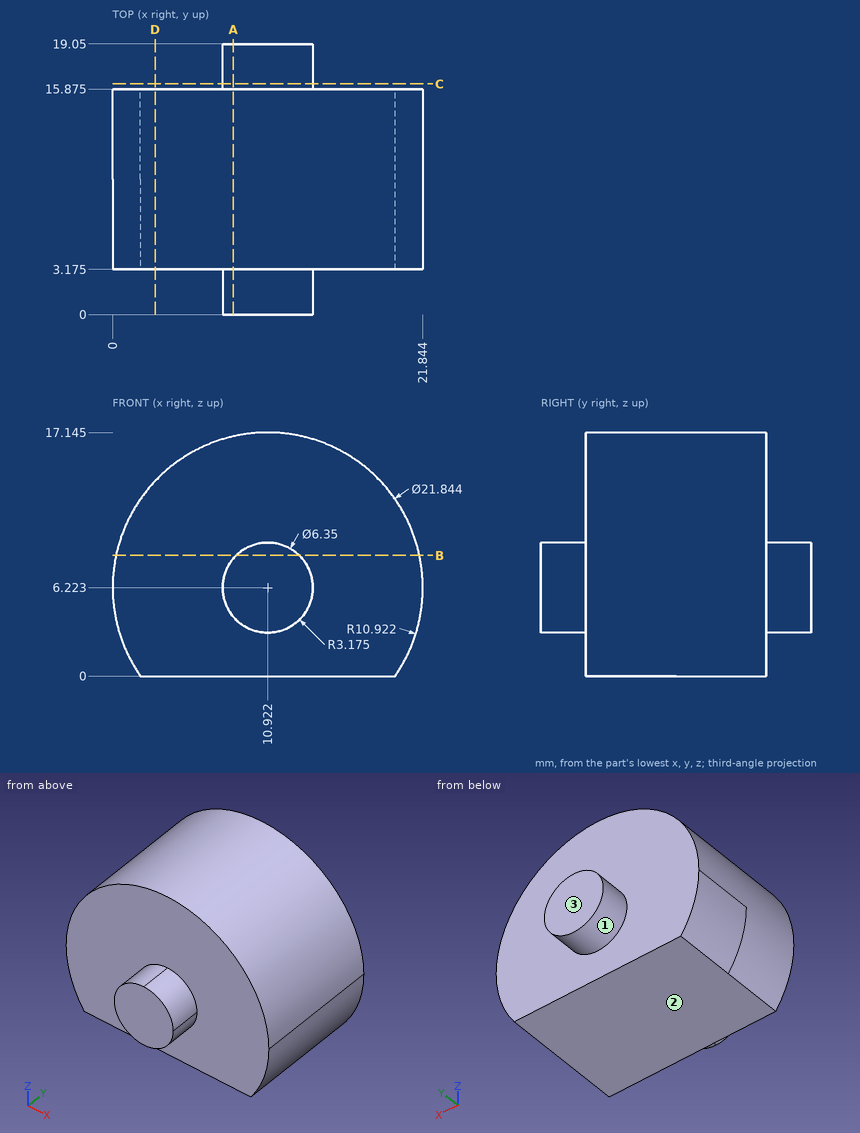
Print and shaded views of the part. All mm, measured from the part's lowest x, y and z. Give positions to 0.01 mm unless a question says otherwise; leave off trailing zeros. Write each loop counter-clockwise with the first axis right and the second up, starting at its lowest first coordinate (ties: lowest second). Pieces come first, ordered by that corner, then holes. Notation, with made-up numbers: (81, 86.5) - (122, 86.5) arc R19 cw to (122, 103.5) - close; hole circle Ø11 at (-33.5, 9.25). An arc over 180 degrees is marked (long way). One line per question, with ' | ' between items. Start each with the question number.
(1) Slice it at B-B on z = 8.5. Write the cut outline in (x, y) (3 decimals), plus the area to 3 significant figures.
(2) Slice it at D-D on x = 3. Write the cut outline in (y, z) (3 decimals), plus the area to 3 significant figures.
(3) Two-plate mould, pull along Z, no slides. Class the marked faces 1, 2 and 3: +Z half, -Z half, draft (parallel to the pull), parting line (faces both ways), or undercut.
(4) Slice it at C-C on y = 16.25. Write the cut outline in (x, z) (3 decimals), plus the area to 3 significant figures.
(5) Wall check: line 1 along Y through (x, z) = (1, 8.75) (3 decimals); line 2 along X through (y, z) = (6.75, 8.5); line 3 along Z through (x, y) = (2.5, 14.25). Give the ranges that are in metal, low to high. Write a range as from..to.
(6) Pin check, flat tips, straight feed: P1, Ø1.5, axis at x = 2.5, z = 10.5, coming from the -Y side (3 decimals); P2, Ø8, axis at x = 6, y = 8.5, coming from the +Z side. Stop position of each tip, or through.
(7) Slice it at A-A on x = 8.5. Write the cut outline in (y, z) (3 decimals).
Results below:
1) outline: (0.24, 3.175) - (8.709, 3.175) - (8.709, 0) - (13.135, 0) - (13.135, 3.175) - (21.604, 3.175) - (21.604, 15.875) - (13.135, 15.875) - (13.135, 19.05) - (8.709, 19.05) - (8.709, 15.875) - (0.24, 15.875) - close | area: 299 mm^2
2) outline: (3.175, 0) - (15.875, 0) - (15.875, 13.742) - (3.175, 13.742) - close | area: 175 mm^2
3) face 1: parting line | face 2: -Z half | face 3: draft
4) outline: circle Ø6.35 at (10.922, 6.223) | area: 31.7 mm^2
5) line 1: 3.175..15.875 | line 2: 0.24..21.6 | line 3: 0..13.18
6) P1: y = 3.175 | P2: z = 17.11
7) outline: (0, 4.17) - (3.175, 4.17) - (3.175, 0) - (15.875, 0) - (15.875, 4.17) - (19.05, 4.17) - (19.05, 8.276) - (15.875, 8.276) - (15.875, 16.873) - (3.175, 16.873) - (3.175, 8.276) - (0, 8.276) - close
